Source: CAD feature listing. Evaluate the final solid. Frame: model axes, mm. Round coordinates to 2 decimals unless told otherwise and drop trailing zeros. One line per item, written item: value.
Autodesk Inventor part; units mm, degrees
ref_plane "YZ Plane" through (0, 0, 0) normal (1, 0, 0) x (0, 1, 0)
ref_plane "XZ Plane" through (0, 0, 0) normal (0, 1, 0) x (-1, 0, 0)
ref_plane "XY Plane" through (0, 0, 0) normal (0, 0, 1) x (1, 0, 0)
sketch "Sketch1" plane through (0, 0, 0) normal (1, 0, 0) x (0, 1, 0)
  line L0 (-12.7, 180) -> (12.7, 180)
  line L1 (12.7, 180) -> (12.7, -180)
  line L2 (12.7, -180) -> (-12.7, -180)
  line L3 (-12.7, -180) -> (-12.7, 180)
  line L4 (-12.7, 180) -> (12.7, -180) construction
  line L5 (12.7, 180) -> (-12.7, -180) construction
  point P0 (0, 0)
  dimension "d0" = 25.4
  dimension "d1" = 360
extrude "Extrusion1" add sketch "Sketch1" along normal blind 3.175
sketch "Sketch2" plane through (3.175, 0, 0) normal (1, 0, 0) x (0, 0, -1)
  line L0 (180, -12.7) -> (180, 12.7)
  line L1 (180, 12.7) -> (-180, 12.7)
  line L2 (-180, 12.7) -> (-180, -12.7)
  line L3 (-180, -12.7) -> (180, -12.7)
  circle A0 centre (-168, -1.68) radius 2.5
  line L4 (180, 12.7) -> (-180, 12.7)
  line L5 (0, 12.7) -> (0, -12.7)
  circle A1 centre (168, -1.68) radius 2.5
  circle A2 centre (-154.6, -1.68) radius 2.5
  circle A3 centre (154.6, -1.68) radius 2.5
  point P0 (0, 0)
  dimension "d4" = 5
  dimension "d5" = 14.38
  dimension "d6" = 12
  dimension "d9" = 13.4
extrude "Extrusion2" cut sketch "Sketch2" against normal through all contours A0 | A1 | A2 | A3
sketch "Sketch3" plane through (3.175, 0, 0) normal (1, 0, 0) x (0, 0, -1)
  circle A0 centre (-168, -1.68) radius 2.5
  circle A1 centre (154.6, -1.68) radius 2.5
  circle A2 centre (168, -1.68) radius 2.5
  circle A3 centre (-154.6, -1.68) radius 2.5
  line L0 (180, -12.7) -> (180, 12.7)
  line L1 (180, 12.7) -> (-180, 12.7)
  line L2 (-180, 12.7) -> (-180, -12.7)
  line L3 (-180, -12.7) -> (180, -12.7)
  circle A4 centre (-168, -1.68) radius 2.5
  circle A5 centre (-154.6, -1.68) radius 2.5
  circle A6 centre (-48, -1.68) radius 2.5
  circle A7 centre (-34.6, -1.68) radius 2.5
  line L4 (0, 0) -> (0, 12.7)
  circle A8 centre (48, -1.68) radius 2.5
  circle A9 centre (34.6, -1.68) radius 2.5
  dimension "d12" = 120
extrude "Extrusion3" cut sketch "Sketch3" against normal through all contours A6 | A7 | A8 | A9
properties part number "PLENTINA_CANALETA_MOVIL" material "Steel, Mild, Welded"
1. Ray query, line 1 (Y direction, x = 2.4, z = -34.6). Return the intervals inside material, ascending. Write a range as [from, to].
Report:
line 1: y = [-12.7, -4.18], [0.82, 12.7]
2. Section query A-A (x = 2.1). Count the separate pieces of the cut face and the enclosed holes in it, and give its area (3 significant figures).
Report:
separate pieces: 1
enclosed holes: 8
area: 8,990 mm2
3. Pin query (flat end, axial travel): pin 1 (4 mm diameter, centred on y = -1.68, z = 168, fed in from -X); pin 2 (8 mm diameter, centred on y = -1.68, z = -168, fed in from +X) (3 decimals). Return the tip coordinate at first contact, or that it passes through.
Report:
pin 1: passes through
pin 2: stops at x = 3.175
